The drawing under review shows one solid part. Ordinate dimensions are in mm from its lowest x, y, z. A direction names the side the tool comes from. Round coordinates to 2 decimals unless told otherwise and drop trailing zeros. Order: outer loops, then holes, each group sorted by start corner. A loop starts at its lowest first (then second) coordinate and runs counter-clockwise, first axis right, second up. Notation, with made-up numbers: M 44.5,82.5 L 78.5,82.5 A19 cw 78.5,117.5 Z; hole C 53.5,49 d2. An arc over 180 degrees is marked long. Answer as a JSON object with one key per item and string values. Group by question number.
1. Clearance check with flat-ended pins moving along their axes: P1, Ø8, axis at y = 134.5, z = 25, coming from the +X side; P2, Ø12, axis at x = 11, z = 21.5, coming from the -Y side; P3, Ø16.5, axis at x = 9, z = 19.5, coming from the +Y side. State where each tip first meets the part, or that it passes through.
2. To check wall thickness, follow probe 1 along X at (y, z) = (78, 22); probe 2 along Z at (x, y) = (117, 69.5); probe 3 along Y at (x, z) = (112.5, 6). State the ranges of each line that lie inside material, in increasing order. Write a range as [from, to].
3. Add section A-A on z = 22.5. State the section outline as (x, y) points.
4. Mouldability with a two-part tool opening along Y and no side actions: class the marked faces 3, 4 and 5 as released by +Y, released by -Y, zero draft, split by the parting line, or undercut.
5. Machinability: for the marked faces 1 and 2, which of the approach directions +Z, -Z, +X, -X, +Y, -Y give a long, thin tool a straight path to every point of the face, cutting with its end or side? Answer none if there is none.
6. Add section B-B on z = 12.5. State the section outline as (x, y) points, and give its area (3 significant figures).
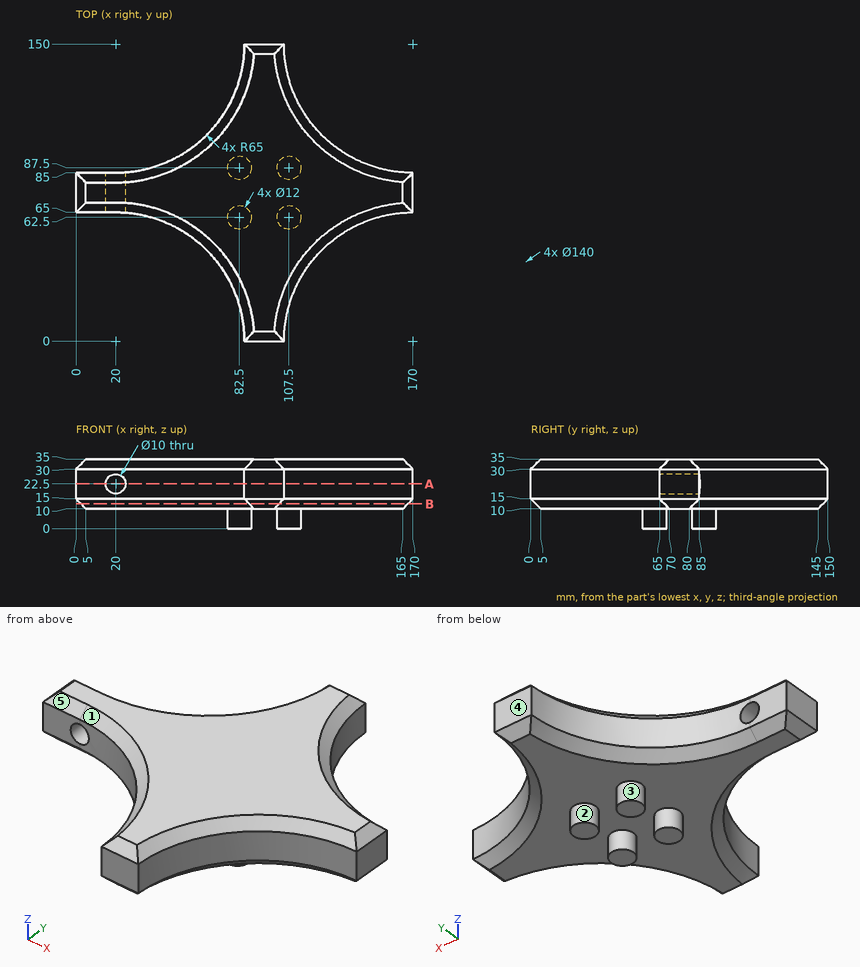
Recorded:
{
 "1": {"P1": "stops at x = 107.99", "P2": "stops at y = 65", "P3": "stops at y = 85"},
 "2": {"probe 1": "x = [0, 15.03], [24.97, 170]", "probe 2": "z = [10, 35]", "probe 3": "y = [59.18, 65.82], [84.18, 90.82]"},
 "3": {"outline": "M 0,65 L 15,65 L 15,85 L 0,85 Z; M 25,64.81 A65 cw 85,0 L 105,0 A65 cw 170,65 L 170,85 A65 cw 105,150 L 85,150 A65 cw 25,85.19 Z"},
 "4": {"face 3": "undercut", "face 4": "released by +Y", "face 5": "released by -Y"},
 "5": {"face 1": "+Z, -X, -Y", "face 2": "-Z"},
 "6": {"outline": "M 2.5,67.5 L 20,67.5 A67.5 cw 87.45,2.5 L 102.55,2.5 A67.5 cw 167.5,67.45 L 167.5,82.55 A67.5 cw 102.55,147.5 L 87.45,147.5 A67.5 cw 20,82.5 L 2.5,82.5 Z", "area": "8,340 mm²"}
}
